The figure shows three views and two pictorial views of one solid part (mm, origin at its lowest corner). Answer the questions. A direction names the side the tool comes from. Give positions to 0.01 mm unless a question says otherwise; leave off trailing zeros. Loops run counter-clockwise (first coordinate to the right, second up) from the corner with the lowest first, then second, coordinate; pieces in that order, holes last. Notation, with made-up numbers: (52, 15) - (77, 15) arc R12 cw to (77, 25) - close; hole circle Ø2 at (40.25, 24.5). An arc over 180 degrees is marked (long way). One line per question, with ' | ' between items.
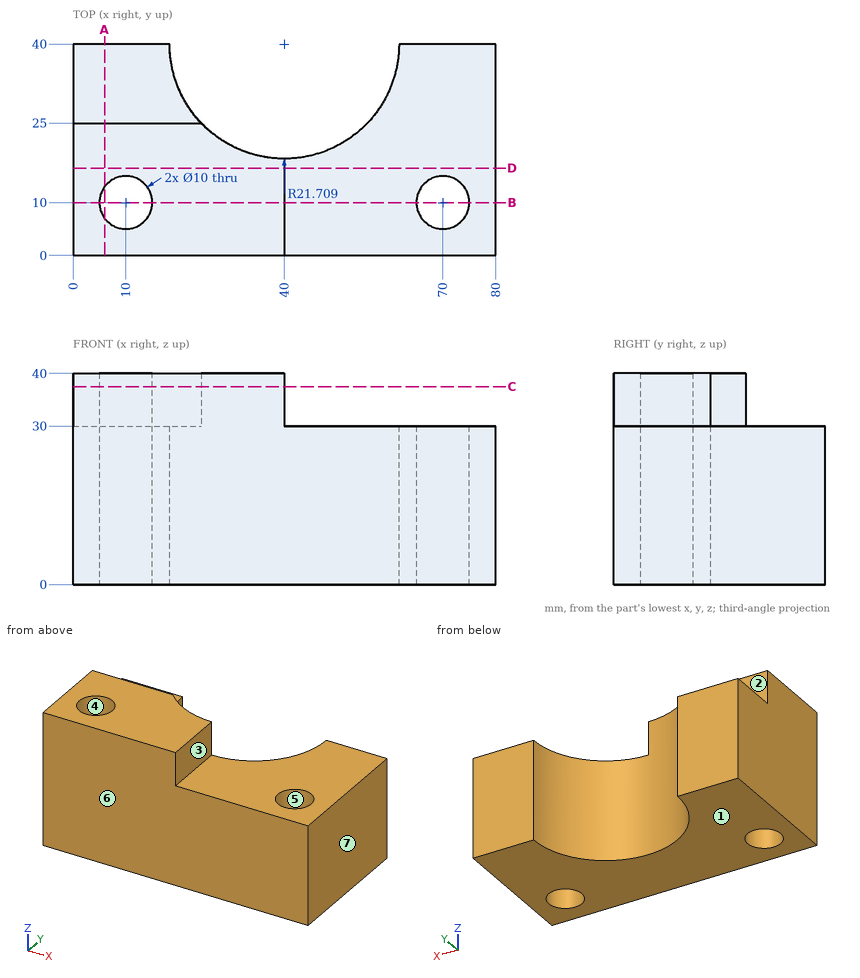
1. Which of the six approach directions +Z, -Z, +X, -X, +Y, -Y give full straight-line access (tool end or side, diameter ignored) to the marked faces 1, 2 and 3?
Evaluation:
face 1: -Z, +X, -X, +Y, -Y | face 2: +Z, +X, -X, +Y | face 3: +Z, +X, +Y, -Y
2. Find section A-A on x = 6. Write down the section's boundary in (y, z), then the cut area to 3 significant figures.
Evaluation:
outline: (0, 0) - (7, 0) - (7, 40) - (0, 40) - close; (13, 0) - (40, 0) - (40, 30) - (25, 30) - (25, 40) - (13, 40) - close | area: 1,210 mm2
3. Flat-ended cylindrical pins translate along their axes: pin 1 (3 mm diameter, centred on y = 9, z = 37.5, fed in from +X); pin 2 (4 mm diameter, centred on x = 47, z = 19.5, fed in from +Y) (1 decimal); pin 3 (4.5 mm diameter, centred on x = 6.5, y = 29.5, fed in from +Z). Find the tip coordinate at first contact, or state that the pin passes through.
Evaluation:
pin 1: x = 40 | pin 2: y = 20.2 | pin 3: z = 30
4. Consider L1, parallel to Y at x = 10, z = 28.5; L2, parallel to Z at x = 71.5, y = 5; L3, parallel to Y at x = 12, z = 25. Determine where each line is inside the solid, lowest interval first.
Evaluation:
L1: 0 to 5, 15 to 40 | L2: 0 to 30 | L3: 0 to 5.42, 14.58 to 40
5. Find section C-C on z = 37.5. Write down the section's boundary in (x, y), then the cut area to 3 significant figures.
Evaluation:
outline: (0, 0) - (40, 0) - (40, 18.29) arc R21.71 cw to (24.31, 25) - (0, 25) - close; hole circle Ø10 at (10, 10) | area: 849 mm2
6. Determine the mould class of the marked faces 4, 5, 6 and 7 for opening direction Y: +Y half, -Y half, draft (parallel to the pull), parting line (faces both ways), or undercut.
Evaluation:
face 4: undercut | face 5: undercut | face 6: -Y half | face 7: draft
7. Find section B-B on y = 10. Write down the section's boundary in (x, z), then the cut area to 3 significant figures.
Evaluation:
outline: (0, 0) - (5, 0) - (5, 40) - (0, 40) - close; (15, 0) - (65, 0) - (65, 30) - (40, 30) - (40, 40) - (15, 40) - close; (75, 0) - (80, 0) - (80, 30) - (75, 30) - close | area: 2,100 mm2
8. Find section D-D on y = 16.5. Write down the section's boundary in (x, z), then the cut area to 3 significant figures.
Evaluation:
outline: (0, 0) - (80, 0) - (80, 30) - (40, 30) - (40, 40) - (0, 40) - close | area: 2,800 mm2
